Build history of the part. All positions in model axes, mm. Give positions to 0.01 mm unless a question says otherwise; leave off trailing zeros. Write each loop counter-clockwise with the first axis right and the second up, starting at its lowest first coordinate (ties: lowest second). Pieces come first, ordered by that corner, then holes. Notation, with made-up numbers: M 10,74.25 L 42,74.25 A23 ccw 42,90.25 Z; hole C -27.5,17.5 d5. An arc over 180 degrees is marked long. One line per item, written item: value. Start each with the question number.
from build123d import *

# Parameters (mm, degrees)
F0_W     = 541.782
F0_H     = 50.8
F0_W_2   = 541.7734120522
F0_H_2   = 0.0195167541
F0_W_3   = 541.7015288506
F0_H_3   = 0.0952444553
F0_W_4   = 0.0085879478
F0_W_5   = 0.0804711494
F0_H_4   = 50.6215176582
F0_H_5   = 0.1784823418
F0_H_6   = 0.077184248
F0_H_7   = 50.722815752
F1_DEPTH = 3.175


with BuildPart() as f1:
    # F0 (on Top) → F1 (new body)
    with BuildSketch(Plane.XY):
        Polygon((-321.8265879478, -279.4), (-270.891, -279.4), (270.891, -279.4), (321.8984711494, -279.4), (321.8984711494, -279.3047555447), (863.6, -279.3047555447), (863.6, 279.4), (863.5880243454, 279.4), (863.5880243454, 279.322815752), (321.8060243454, 279.322815752), (321.8060243454, 279.4), (270.891, 279.4), (-270.891, 279.4), (-321.623693737, 279.4), (-321.623693737, 279.2215176582), (-863.405693737, 279.2215176582), (-863.405693737, 279.4), (-863.6, 279.4), (-863.6, -279.3804832459), (-321.8265879478, -279.3804832459), align=None)
        with Locations((0, -304.8)):
            Rectangle(F0_W, F0_H)
        Polygon((-321.8265879478, -330.1804832459), (-321.8265879478, -279.4), (-863.6, -279.4), (-863.6085879478, -279.4), (-863.6085879478, -330.1804832459), align=None)
        with Locations((-592.7132939739, -279.3902416229)):
            Rectangle(F0_W_2, F0_H_2)
        with Locations((592.7492355747, -279.3523777723)):
            Rectangle(F0_W_3, F0_H_3)
        Polygon((863.6, -279.4), (321.8984711494, -279.4), (321.8984711494, -330.1047555447), (863.6804711494, -330.1047555447), (863.6804711494, -279.4), align=None)
        with Locations((-863.6042939739, -279.3902416229)):
            Rectangle(F0_W_4, F0_H_2)
        with Locations((863.6402355747, -279.3523777723)):
            Rectangle(F0_W_5, F0_H_3)
        Polygon((-863.6085879478, -279.3804832459), (-863.6, -279.3804832459), (-863.6, 279.4), (-914.4, 279.4), (-914.4, -279.4), (-863.6085879478, -279.4), align=None)
        Polygon((863.6, 279.4), (863.6, -279.3047555447), (863.6804711494, -279.3047555447), (863.6804711494, -279.4), (914.4, -279.4), (914.4, 279.4), align=None)
        with Locations((-592.514693737, 304.7107588291)):
            Rectangle(F0_W, F0_H_4)
        with Locations((-592.514693737, 279.3107588291)):
            Rectangle(F0_W, F0_H_5)
        with Locations((592.6970243454, 279.361407876)):
            Rectangle(F0_W, F0_H_6)
        with Locations((592.6970243454, 304.761407876)):
            Rectangle(F0_W, F0_H_7)
        with Locations((0, 304.8)):
            Rectangle(F0_W, F0_H)
    extrude(amount=F1_DEPTH)


solid = f1.part
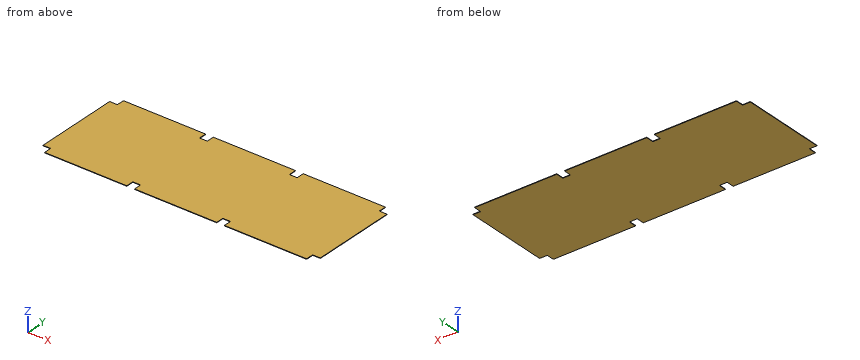
1) Band-saw the part on A-A (z = 1.35). List the corners of the cut face in (x, y), then the cut area to 3 significant figures.
2) Probe line 1 along X through (y, z) = (-300, 0.25); line 2 along X through (y, z) = (285, 2.9); line 3 along Y through (x, z) = (-571, 1.5). List the from-to ranges inside material, lowest first. Write a range as from..to.
3) Drop flat-ended pins along their axis: P1, Ø1.6, axis at y = -316, z = 1.5, coming from the -X side; P2, Ø1, axis at x = 424.5, y = -230.5, coming from the -Z side; P3, Ø1.6, axis at x = -302.5, z = 2, coming from the -Y side; P4, Ø1, axis at y = 309.5, z = 2, coming from the +X side. Give the stop position or say it passes through.
Model answer:
1. outline: M -914.4,-279.4 L -863.61,-279.4 L -863.61,-330.18 L -321.83,-330.18 L -321.83,-279.4 L -270.89,-279.4 L -270.89,-330.2 L 270.89,-330.2 L 270.89,-279.4 L 321.9,-279.4 L 321.9,-330.1 L 863.68,-330.1 L 863.68,-279.4 L 914.4,-279.4 L 914.4,279.4 L 863.59,279.4 L 863.59,330.12 L 321.81,330.12 L 321.81,279.4 L 270.89,279.4 L 270.89,330.2 L -270.89,330.2 L -270.89,279.4 L -321.62,279.4 L -321.62,330.02 L -863.41,330.02 L -863.41,279.4 L -914.4,279.4 Z
1. area: 1,190,000 mm²
2. line 1: x = -863.61..-321.83, -270.89..270.89, 321.9..863.68
2. line 2: x = -863.41..-321.62, -270.89..270.89, 321.81..863.59
2. line 3: y = -330.18..330.02
3. P1: stops at x = -863.61
3. P2: stops at z = 0
3. P3: stops at y = -279.4
3. P4: stops at x = 863.59
